Part model, mm, in its own coordinate system. Round coordinates to 2 decimals unless told otherwise and drop trailing zeros. Write each loop counter-clockwise with the first axis right and the second up, starting at its lowest first coordinate (ties: lowest second). Pieces come first, ordered by that corner, then holes.
1) Flat gauge pins, fed straight in: pin 1 (4 mm diameter, centred on y = 435, z = 8.5, fed in from +X); pin 2 (1 mm diameter, centred on x = 116, z = 3, fed in from +Y); pin 3 (2 mm diameter, centred on y = 260, z = 7, fed in from +X). Where does each tip first touch, or does it go through?
2) Drill centre lines: L1, parallel to X at y = 357.5, z = 6; L2, parallel to X at y = 408.5, z = 2.25; L3, parallel to Y at x = 117.5, z = 4. Where is each one in solid material? Low to high.
3) Saw through at C-C on y = 363.5. Write the cut outline in (x, z), and give its area (3 significant figures).
4) Saw through at B-B on x = 213. Write the cut outline in (y, z).
5) Saw through at A-A on z = 6.25. Write the cut outline in (x, y).
```python
from build123d import *

# Parameters (mm, degrees)
BOSS_EXTRU_1_DEPTH = 10


with BuildPart() as part:
    # Esquisse1 → Boss.-Extru.1 (new body)
    with BuildSketch(Plane.XY):
        with BuildLine():
            Line((0, 0), (0, 550))
            Line((0, 550), (129.062590026, 604.250037842))
            ThreePointArc((129.062590026, 604.250037842), (144.369719008, 604.329896284), (155.249962158, 593.562590026))
            Line((155.249962158, 593.562590026), (190.859025666, 508.847479263))
            ThreePointArc((190.859025666, 508.847479263), (192.366539865, 502.580756708), (191.802553764, 496.159983364))
            ThreePointArc((191.802553764, 496.159983364), (189.838676364, 331.953031603), (263.189381841, 185.026336182))
            ThreePointArc((263.189381841, 185.026336182), (300.928689878, 157.28521303), (347.160451012, 149.771921656))
            Line((347.160451012, 149.771921656), (422.849515254, 155.480705177))
            ThreePointArc((422.849515254, 155.480705177), (440.508345068, 147.328376864), (442.889156647, 128.024841862))
            Line((442.889156647, 128.024841862), (391, 0))
            Line((391, 0), (0, 0))
        make_face()
    extrude(amount=BOSS_EXTRU_1_DEPTH)


solid = part.part
```
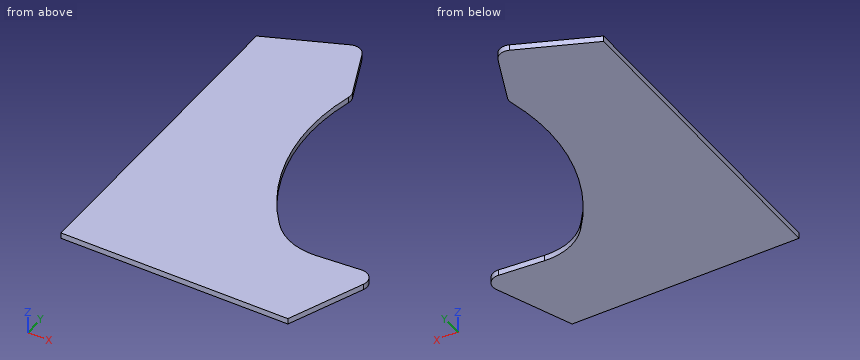
Completed:
1. pin 1: stops at x = 182.05
1. pin 2: stops at y = 598.97
1. pin 3: stops at x = 215.36
2. L1: x = 0 to 184.97
2. L2: x = 0 to 181
2. L3: y = 0 to 599.39
3. outline: (0, 0) - (184.11, 0) - (184.11, 10) - (0, 10) - close
3. area: 1,840 mm2
4. outline: (0, 0) - (264.01, 0) - (264.01, 10) - (0, 10) - close
5. outline: (0, 0) - (391, 0) - (442.89, 128.02) arc R20 ccw to (422.85, 155.48) - (347.16, 149.77) arc R100 cw to (263.19, 185.03) arc R349 cw to (191.8, 496.16) arc R20 ccw to (190.86, 508.85) - (155.25, 593.56) arc R20 ccw to (129.06, 604.25) - (0, 550) - close
